```python
from build123d import *

# Parameters (mm, degrees)
CUT_EXTRUDE1_DEPTH      = 395.646626743
CUT_EXTRUDE1_DEPTH_BACK = 395.646626743
SKETCH2_W               = 193.8
SKETCH2_H               = 31.1
HOLE1_D                 = 12.5


with BuildPart() as part:
    # Sketch1 → Revolve1 (revolve)
    with BuildSketch(Plane.XY, mode=Mode.PRIVATE) as revolve1_sk:
        Polygon((0, 0), (0, 20), (28.9, 20), (28.9, 28), (118.2, 28), (118.2, 43.6), (142.2, 43.6), (142.2, 28), (389.8, 28), (389.8, 0), align=None)
    revolve(revolve1_sk.sketch.rotate(Axis((389.8, 0, 0), (-1, 0, 0)), 90), axis=Axis((389.8, 0, 0), (-1, 0, 0)))

    # Sketch2 → Cut-Extrude1 (cut, two sides: drawn at the far end of the back side and taken through both)
    with BuildSketch(Plane.XY.offset(-CUT_EXTRUDE1_DEPTH_BACK)):
        with Locations((277.8, 12.45)):
            Rectangle(SKETCH2_W, SKETCH2_H)
    extrude(amount=CUT_EXTRUDE1_DEPTH + CUT_EXTRUDE1_DEPTH_BACK, mode=Mode.SUBTRACT)

    # Hole1 (through all)
    with Locations(Plane(origin=(0, -3.1, 0), x_dir=(1, 0, 0), z_dir=(0, 1, 0))):
        with Locations((227.8, 0), (327.8, 0)):
            Hole(HOLE1_D / 2)


solid = part.part
```
Geometry check sheet. Reference: the model listing, model coordinates, mm. A direction names the side the tool comes from. Give positions to 0.01 mm unless a question says otherwise; leave off trailing zeros. Order: outer loops, then holes, each group sorted by start corner. A loop starts at its lowest first (then second) coordinate and runs counter-clockwise, first axis right, second up. Notation, with made-up numbers: (-30.75, -33.5) - (8.25, -33.5) arc R13 cw to (8.25, -14.5) - close; hole circle Ø4 at (53.5, -37). An arc over 180 degrees is marked (long way). Answer in a Markdown table with one row per item. Add a question column.
Q1. Cross-section at A-A, the plane z = 0. Enter the section's corners in (x, y).
Q2. Cross-section at D-D, the plane x = 301.5. Enter the section's corners in (y, z).
Q3. Mould release check, pull along X, two halves, no side actions. Record for faces 1 (the cylindrical face through (322.027, -15.731, 2.394)), 2 (the flat face through (0, 0, 0)), 3 (the flat face through (142.2, 28.5, 0.6)), 4 (the flat face through (180.9, 9, 0)): pulls with the +X half, pulls with the -X half, needs draft (parallel to the pull), parting line crosses it, or undercut.
Q4. Tool access check on faces 5 (the cylindrical face through (267.73, -23.61, -15.05)), 6 (the cylindrical face through (14.65, -0.88, 19.98)), 7 (the flat face through (276, -3.1, 0)). Record the directions out of +Z, -Z, +X, -X, +Y, -Y that give a thin tool (end or side, any length) a straight path to the whole face; none if there is none.
Q5. Material ranges on probe 1 along X at (y, z) = (8.5, -3.5); probe 2 along Y at (x, z) = (366.5, 0); probe 3 along X at (y, z) = (-22, -34), recorded low to high. Write a range as from..to.
Q6. Gauge pin test, flat ends, axial feed: pin 1 (16 mm diameter, centred on x = 327.8, z = 0, fed in from +Y); pin 2 (4 mm diameter, centred on x = 113, y = 21.5, fed in from +Z); pin 3 (8 mm diameter, centred on y = 1, z = -30.5, fed in from -X); pin 4 (7.5 mm diameter, centred on x = 227.8, z = 0, fed in from -Y). Record the tip position at first contact, or that the pin passes through.
Q7. Cross-section at C-C, the plane x = 227.8. Enter the section's corners in (y, z), then the cut area to 3 significant figures.
Q8. Cross-section at B-B, the plane y = 4.5. Enter the section's corners in (x, z), then the cut area to 3 significant figures.
Check values:
| question | item | result |
|---|---|---|
| 1 | outline | (0, -20) - (28.9, -20) - (28.9, -28) - (118.2, -28) - (118.2, -43.6) - (142.2, -43.6) - (142.2, -28) - (221.55, -28) - (221.55, -3.1) - (180.9, -3.1) - (180.9, 28) - (142.2, 28) - (142.2, 43.6) - (118.2, 43.6) - (118.2, 28) - (28.9, 28) - (28.9, 20) - (0, 20) - close; (234.05, -28) - (321.55, -28) - (321.55, -3.1) - (234.05, -3.1) - close; (334.05, -28) - (389.8, -28) - (389.8, 28) - (374.7, 28) - (374.7, -3.1) - (334.05, -3.1) - close |
| 2 | outline | (-3.1, -27.83) - (-3.1, 27.83) arc R28 ccw to start |
| 3 | face 1 | undercut |
| 3 | face 2 | pulls with the -X half |
| 3 | face 3 | pulls with the +X half |
| 3 | face 4 | undercut |
| 4 | face 5 | +X |
| 4 | face 6 | -X |
| 4 | face 7 | +Z, -Z, +Y |
| 5 | probe 1 | x = 0..180.9, 374.7..389.8 |
| 5 | probe 2 | y = -28..-3.1 |
| 5 | probe 3 | x = 118.2..142.2 |
| 6 | pin 1 | stops at y = -3.1 |
| 6 | pin 2 | stops at z = 20.09 |
| 6 | pin 3 | stops at x = 28.9 |
| 6 | pin 4 | passes through |
| 7 | outline | (-27.29, -6.25) arc R28 ccw to (-3.1, -27.83) - (-3.1, -6.25) - close; (-27.29, 6.25) - (-3.1, 6.25) - (-3.1, 27.83) arc R28 ccw to start |
| 7 | area | 750 mm^2 |
| 8 | outline | (0, -19.49) - (28.9, -19.49) - (28.9, -27.64) - (118.2, -27.64) - (118.2, -43.37) - (142.2, -43.37) - (142.2, -27.64) - (180.9, -27.64) - (180.9, 27.64) - (142.2, 27.64) - (142.2, 43.37) - (118.2, 43.37) - (118.2, 27.64) - (28.9, 27.64) - (28.9, 19.49) - (0, 19.49) - close; (374.7, -27.64) - (389.8, -27.64) - (389.8, 27.64) - (374.7, 27.64) - close |
| 8 | area | 11,100 mm^2 |
